Verification items for the finished model (mm, model axes). A direction names the side the tool comes from. Give positions to 0.01 mm unless a question says otherwise; leave off trailing zeros. Write each loop counter-clockwise with the first axis right and the second up, starting at its lowest first coordinate (ties: lowest second). Pieces come first, ordered by that corner, then holes. Notation, with made-up numbers: (-11, -26.5) -> (44, -26.5) arc R25 ccw to (44, -9.5) -> close; hole circle Ø1 at (60.5, -20). An arc over 180 degrees is marked (long way). Use CSV: the item, a comma, the result in double quotes. Start each with the question number.
```python
from build123d import *
from OCP.BRepFilletAPI import BRepFilletAPI_MakeChamfer

# Parameters (mm, degrees)
RESSALTO_EXTRUS_O1_DEPTH = 18.35
ESBO_O2_R                = 9.25
CORTE_EXTRUS_O1_DEPTH    = 30.058016679
ESBO_O3_R                = 19.09752109
ESBO_O3_R_2              = 12.25
CORTE_EXTRUS_O2_DEPTH    = 7.5
FILETE1_R                = 2
CHANFRO1_SIZE            = 0.5
CHANFRO1_SIZE2           = 0.08816349
FILETE2_R                = 1
CHANFRO3_SIZE            = 2.5
CHANFRO3_SIZE2           = 0.909925586
FILETE3_R                = 1.5


with BuildPart() as part:
    # Esboço1 → Ressalto-extrusão1 (new body)
    with BuildSketch(Plane.XY):
        Polygon((0, -17.031832941), (14.75, -8.515916471), (14.75, 8.515916471), (0, 17.031832941), (-14.75, 8.515916471), (-14.75, -8.515916471), align=None)
    extrude(amount=RESSALTO_EXTRUS_O1_DEPTH)

    # Esboço2 → Corte-extrusão1 (cut, through all)
    with BuildSketch(Plane.XY.offset(18.35)):
        Circle(ESBO_O2_R)
    extrude(amount=-CORTE_EXTRUS_O1_DEPTH, mode=Mode.SUBTRACT)

    # Esboço3 → Corte-extrusão2 (cut)
    with BuildSketch(Plane(origin=(0, 0, 0), x_dir=(-1, 0, 0), z_dir=(0, 0, -1))):
        Circle(ESBO_O3_R)
        Circle(ESBO_O3_R_2, mode=Mode.SUBTRACT)
    extrude(amount=-CORTE_EXTRUS_O2_DEPTH, mode=Mode.SUBTRACT)

    # Filete1
    filete1_edges = [part.edges().sort_by_distance(p)[0] for p in [
        (-9.25, 0, 0),
    ]]
    fillet(filete1_edges, radius=FILETE1_R)

    # Chanfro1: one chamfer whose edges measure the first distance from different faces: ONE call of the kernel's chamfer builder (chamfer() names one face for all edges)
    chanfro1_edges_1 = [part.edges().sort_by_distance(p)[0] for p in [
        (-14.75, 0, 7.5),
    ]]
    chanfro1_side_1 = [part.faces().sort_by_distance(p)[0] for p in [
        (-14.75, 0, 12.925),
    ]]
    chanfro1_edges_2 = [part.edges().sort_by_distance(p)[0] for p in [
        (7.375, -12.773874706, 7.5),
    ]]
    chanfro1_side_2 = [part.faces().sort_by_distance(p)[0] for p in [
        (7.375, -12.773874706, 12.925),
    ]]
    chanfro1_edges_3 = [part.edges().sort_by_distance(p)[0] for p in [
        (-7.375, -12.773874706, 7.5),
    ]]
    chanfro1_side_3 = [part.faces().sort_by_distance(p)[0] for p in [
        (-7.375, -12.773874706, 12.925),
    ]]
    chanfro1_edges_4 = [part.edges().sort_by_distance(p)[0] for p in [
        (-7.375, 12.773874706, 7.5),
    ]]
    chanfro1_side_4 = [part.faces().sort_by_distance(p)[0] for p in [
        (-7.375, 12.773874706, 12.925),
    ]]
    chanfro1_edges_5 = [part.edges().sort_by_distance(p)[0] for p in [
        (7.375, 12.773874706, 7.5),
    ]]
    chanfro1_side_5 = [part.faces().sort_by_distance(p)[0] for p in [
        (7.375, 12.773874706, 12.925),
    ]]
    chanfro1_edges_6 = [part.edges().sort_by_distance(p)[0] for p in [
        (14.75, 0, 7.5),
    ]]
    chanfro1_side_6 = [part.faces().sort_by_distance(p)[0] for p in [
        (14.75, 0, 12.925),
    ]]
    chanfro1 = BRepFilletAPI_MakeChamfer(part.part.solid().wrapped)
    for e in chanfro1_edges_1:
        chanfro1.Add(CHANFRO1_SIZE, CHANFRO1_SIZE2, e.wrapped, chanfro1_side_1[0].wrapped)  # the first distance lies on this face
    for e in chanfro1_edges_2:
        chanfro1.Add(CHANFRO1_SIZE, CHANFRO1_SIZE2, e.wrapped, chanfro1_side_2[0].wrapped)  # the first distance lies on this face
    for e in chanfro1_edges_3:
        chanfro1.Add(CHANFRO1_SIZE, CHANFRO1_SIZE2, e.wrapped, chanfro1_side_3[0].wrapped)  # the first distance lies on this face
    for e in chanfro1_edges_4:
        chanfro1.Add(CHANFRO1_SIZE, CHANFRO1_SIZE2, e.wrapped, chanfro1_side_4[0].wrapped)  # the first distance lies on this face
    for e in chanfro1_edges_5:
        chanfro1.Add(CHANFRO1_SIZE, CHANFRO1_SIZE2, e.wrapped, chanfro1_side_5[0].wrapped)  # the first distance lies on this face
    for e in chanfro1_edges_6:
        chanfro1.Add(CHANFRO1_SIZE, CHANFRO1_SIZE2, e.wrapped, chanfro1_side_6[0].wrapped)  # the first distance lies on this face
    add(Compound.cast(chanfro1.Shape()), mode=Mode.REPLACE)

    # Filete2
    filete2_edges = [part.edges().sort_by_distance(p)[0] for p in [
        (12.25, 0, 7.5),
    ]]
    fillet(filete2_edges, radius=FILETE2_R)

    # Chanfro3
    chanfro3_edges = [part.edges().sort_by_distance(p)[0] for p in [
        (14.75, 0, 18.35),
        (7.375, 12.773874706, 18.35),
        (-7.375, 12.773874706, 18.35),
        (-14.75, 0, 18.35),
        (-7.375, -12.773874706, 18.35),
        (7.375, -12.773874706, 18.35),
    ]]
    chanfro3_side = [part.faces().sort_by_distance(p)[0] for p in [
        (7.149690028, -12.383626387, 18.35),
    ]]
    chamfer(chanfro3_edges, length=CHANFRO3_SIZE, length2=CHANFRO3_SIZE2, reference=chanfro3_side[0])

    # Filete3
    filete3_edges = [part.edges().sort_by_distance(p)[0] for p in [
        (-9.25, 0, 18.35),
    ]]
    fillet(filete3_edges, radius=FILETE3_R)


solid = part.part
```
(1) Thickness scan on line 1 (X direction, y = 4.5, z = 12.75); line 2 (X direction, y = 1, z = 1.5); line 3 (Y direction, x = 8.25, z = 9.5). Record the ranges inside material, lowest first. Write a range as from..to.
(2) Section check A-A on y = 0. Record the cut outline in (x, z).
(3) Set-up check for faces 1 (the face through (6.86, 11.65, 17.89)), 2 (the face through (8, -11, 7.5)): record each of +Z, -Z, +X, -X, +Y, -Y from which the full face is reachable in a straight line by a thin tool's end or side.
(4) Draft check along Y on faces 3 (the face through (13.517, -0.119, 17.889)), 4 (the face through (-2.01, -9.03, 9.53)), 5 (the face through (-7.249, -12.795, 7.746)), 6 (the face through (7.5, 12.7, 12.7)). Enter one of: released by +Y, released by -Y, zero draft, split by the parting line, or undercut.
(5) Section check B-B on z = 5.25. Record the cut outline in (x, y), then the cut area to 3 significant figures.
(6) Go/stop test with flat-tipped pins: pin 1 (14.5 mm diameter, centred on x = 1.5, y = 3, fed in from -Z); pin 2 (3 mm diameter, centred on x = 2.5, z = 14.5, fed in from -Y); pin 3 (10 mm diameter, centred on x = 7, z = 14, fed in from -Y); pin 4 (2 mm diameter, centred on x = 9.5, y = 13.5, fed in from +Z). Record where each tip stops, or that it passes through.
Data:
1,line 1,"x = -14.75..-8.08, 8.08..14.75"
1,line 2,"x = -12.21..-9.26, 9.26..12.21"
1,line 3,"y = -12.27..-4.18, 4.18..12.27"
2,outline,"(-14.75, 8) -> (-14.66, 7.5) -> (-13.25, 7.5) arc R1 cw to (-12.25, 6.5) -> (-12.25, 0) -> (-11.25, 0) arc R2 ccw to (-9.25, 2) -> (-9.25, 16.85) arc R1.5 ccw to (-10.75, 18.35) -> (-12.25, 18.35) -> (-14.75, 17.44) -> close; (9.25, 2) arc R2 ccw to (11.25, 0) -> (12.25, 0) -> (12.25, 6.5) arc R1 cw to (13.25, 7.5) -> (14.66, 7.5) -> (14.75, 8) -> (14.75, 17.44) -> (12.25, 18.35) -> (10.75, 18.35) arc R1.5 ccw to (9.25, 16.85) -> close"
3,face 1,"+Z, +X, +Y"
3,face 2,"-Z"
4,face 3,"zero draft"
4,face 4,"undercut"
4,face 5,"released by -Y"
4,face 6,"released by +Y"
5,outline,"circle Ø24.5 at (0, 0); hole circle Ø18.5 at (0, 0)"
5,area,"203 mm2"
6,pin 1,"stops at z = 0.11"
6,pin 2,"stops at y = -16.45"
6,pin 3,"stops at y = -15.88"
6,pin 4,"passes through"
